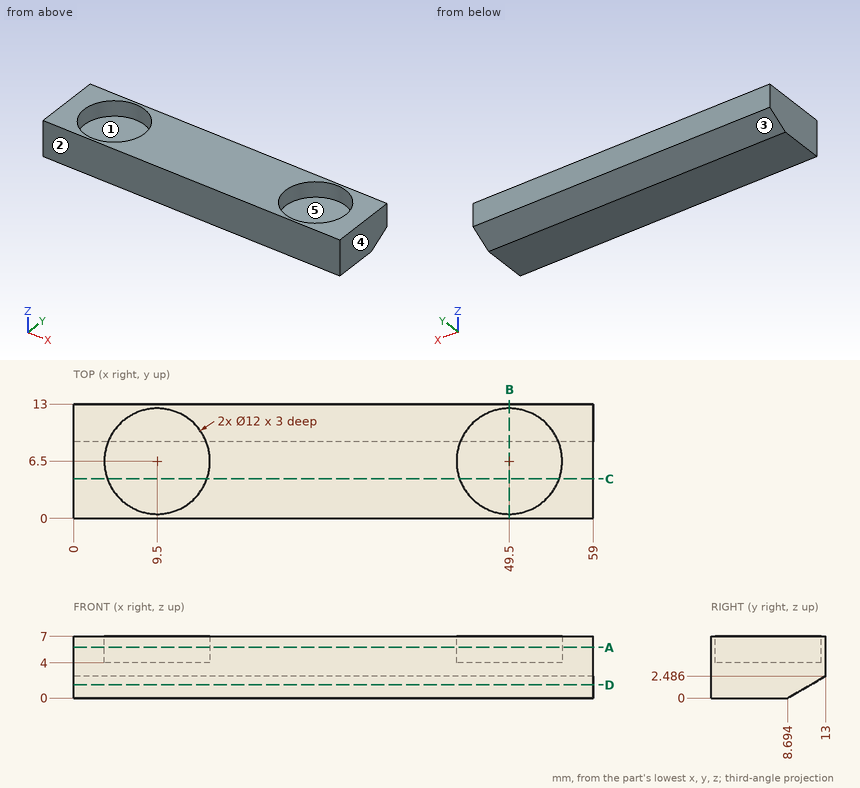
Design review of the part shown in the three views and the two pictorial views. Dimensions are in mm from the part's minimum x, y and z. A direction names the side the tool comes from. Give positions to 0.01 mm unless a question says otherwise; leave off trailing zeros. Loops run counter-clockwise (first coordinate to the right, second up) from the corner with the lowest first, then second, coordinate; pieces in that order, holes last. Notation, with made-up numbers: M -9.75,18 L 36.25,18 A17 cw 36.25,42 Z; hole C 49,-18 d11. An arc over 180 degrees is marked long. Answer as a JSON object with one key per item and string values. Group by question number.
Q1. Add section D-D on z = 1.5. Give the boundary of the cut face in (x, y).
Q2. Insertion check: P1, Ø6, axis at x = 48, y = 8.5, coming from the +Z side; P2, Ø1.5, axis at x = 31, z = 1, coming from the -Y side. Each pin has a flat end and moves straight along its axis. Give the tip position at first contact, or say it passes through.
Q3. Add section C-C on y = 4.5. Give the boundary of the cut face in (x, z), and give its area (3 significant figures).
Q4. Add section B-B on x = 49.5. Give the boundary of the cut face in (y, z).
Q5. Tool access review of the marked faces 1 and 2: name each direction out of +Z, -Z, +X, -X, +Y, -Y from which nothing blocks a thin tool from reaching the whole face with its end or side.
Q6. Add section A-A on z = 5.75. Give the boundary of the cut face in (x, y).
Q7. Mouldability with a two-part tool opening along Y and no side actions: class the marked faces 3, 4 and 5 as +Y half, -Y half, draft (parallel to the pull), parting line (faces both ways), or undercut.
Q8. For probe 1 along Y at (x, z) = (49.5, 5.45); probe 2 along X at (y, z) = (11.5, 5.25); probe 3 along X at (y, z) = (10.75, 6) (1 decimal), list the stretches that pass through material, from the lowest coordinate up. Write a range as [from, to].
Checked values:
{
 "1": {"outline": "M 0,0 L 59,0 L 59,11.29 L 0,11.29 Z"},
 "2": {"P1": "z = 4", "P2": "y = 0"},
 "3": {"outline": "M 0,0 L 59,0 L 59,7 L 55.16,7 L 55.16,4 L 43.84,4 L 43.84,7 L 15.16,7 L 15.16,4 L 3.84,4 L 3.84,7 L 0,7 Z", "area": "345 mm²"},
 "4": {"outline": "M 0,0 L 8.69,0 L 13,2.49 L 13,7 L 12.5,7 L 12.5,4 L 0.5,4 L 0.5,7 L 0,7 Z"},
 "5": {"face 1": "+Z", "face 2": "+Z, -Z, +X, -X, -Y"},
 "6": {"outline": "M 0,0 L 59,0 L 59,13 L 0,13 Z; hole C 9.5,6.5 d12; hole C 49.5,6.5 d12"},
 "7": {"face 3": "+Y half", "face 4": "draft", "face 5": "undercut"},
 "8": {"probe 1": "[0, 0.5], [12.5, 13]", "probe 2": "[0, 6.18], [12.82, 46.18], [52.82, 59]", "probe 3": "[0, 5.3], [13.7, 45.3], [53.7, 59]"}
}
